Here's the drawing with two shaded views (mm, measured from the low corner). I have some questions. A direction names the side the tool comes from. Round coordinates to 2 decimals unless told otherwise and drop trailing zeros. Write each loop counter-clockwise with the first axis right and the second up, starting at its lowest first coordinate (ties: lowest second). Pieces come first, ordered by that corner, then holes.
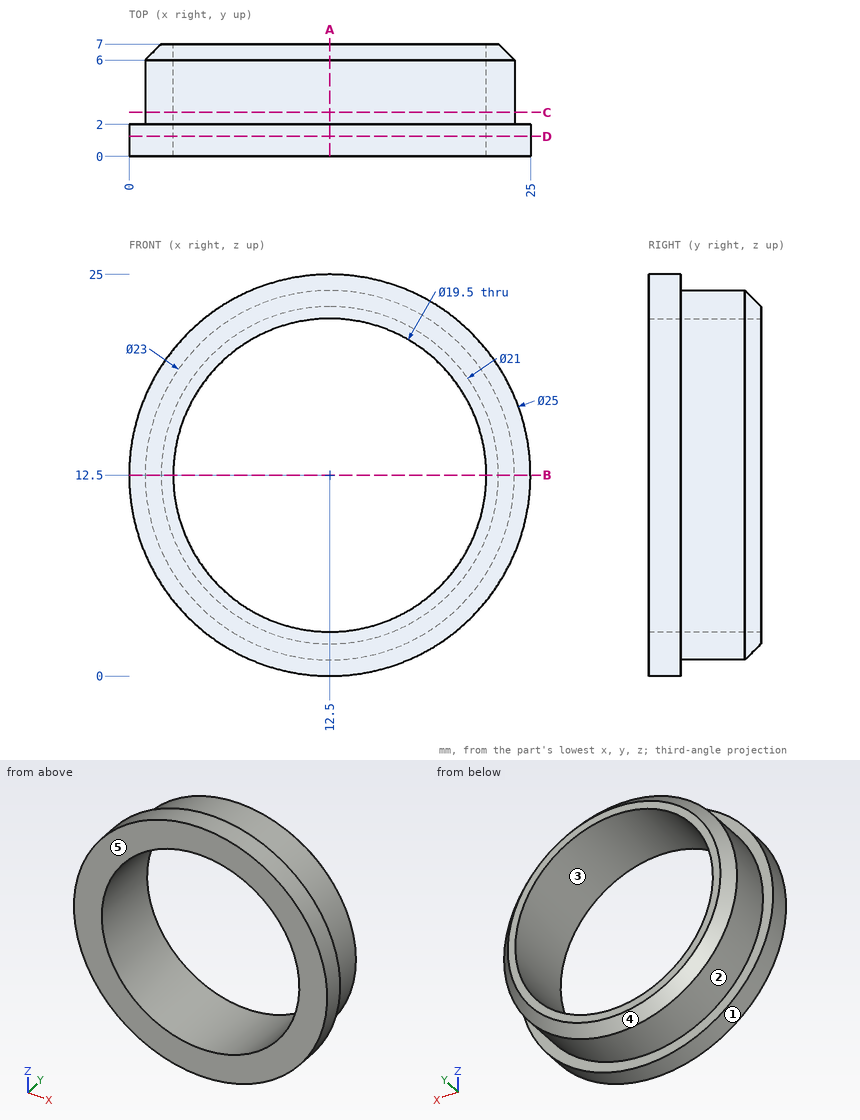
Q1. Imagine slicing it at A-A, the plane x = 12.5. Write out the boundary of the cut face in (y, z).
Q2. If I drill on L1, parallel to Z at x = 12.5, y = 5.25; L2, parallel to X at y = 1.75, z = 12.5; L3, parallel to Y at x = 7, z = 23, over which ranges is the centre line in solid material (lowest first)?
Q3. I'm going to push flat-ended pins straight in: pin 1 Ø3 at (x, y) = (22.5, 3) entering from -Z; pin 2 Ø4 at (x, y) = (16.5, 1) entering from -Z. Where does each tip first touch, or does it pass through?
Q4. On a 3-axis mill with a long thin cutter (end or side, diameter ignored), from which of +Z, -Z, +X, -X, +Y, -Y can I reach the whole of each face in a straight line? I mean the marked faces 1 and 2. Say none if no direction works.
Q5. Imagine slicing it at D-D, the plane y = 1.25. Write out the boundary of the cut face in (x, z).
Q6. Imagine slicing it at B-B, the plane z = 12.5. Write out the boundary of the cut face in (x, y), then the cut area to 3 significant figures.
Q7. Imagine slicing it at C-C, the plane y = 2.75. Write out the boundary of the cut face in (x, z).
Q8. We'd pull the mould along X, two halves only. Please class the marked faces 3, 4 and 5: pulls with the +X half, pulls with the -X half, needs draft (parallel to the pull), parting line crosses it, or undercut.
Results found:
1. outline: (0, 0) - (2, 0) - (2, 1) - (6, 1) - (7, 2) - (7, 2.75) - (0, 2.75) - close; (0, 22.25) - (7, 22.25) - (7, 23) - (6, 24) - (2, 24) - (2, 25) - (0, 25) - close
2. L1: z = 1 to 2.75, 22.25 to 24
2. L2: x = 0 to 2.75, 22.25 to 25
2. L3: y = 0 to 2
3. pin 1: stops at z = 3.7
3. pin 2: stops at z = 0.16
4. face 1: +Y, -Y
4. face 2: +Y
5. outline: circle Ø25 at (12.5, 12.5); hole circle Ø19.5 at (12.5, 12.5)
6. outline: (0, 0) - (2.75, 0) - (2.75, 7) - (2, 7) - (1, 6) - (1, 2) - (0, 2) - close; (22.25, 0) - (25, 0) - (25, 2) - (24, 2) - (24, 6) - (23, 7) - (22.25, 7) - close
6. area: 27.5 mm2
7. outline: circle Ø23 at (12.5, 12.5); hole circle Ø19.5 at (12.5, 12.5)
8. face 3: undercut
8. face 4: parting line crosses it
8. face 5: needs draft
